Design review of the part built by this model. Coordinates are the model's own, in mm. A direction names the side the tool comes from. Coordinates: 2 decimals unless noted, no trailing zeros. Order: outer loops, then holes, each group sorted by start corner. A loop starts at its lowest first (then second) coordinate and runs counter-clockwise, first axis right, second up. Notation, with made-up numbers: M -16,13.5 L -7,13.5 A29 ccw -7,34.5 Z; hole C 57,63.25 d4. An arc over 180 degrees is marked long. Answer as a JSON object with one key per item and string values.
from build123d import *

# Parameters (mm, degrees)
SKETCH_1_W          = 60
SKETCH_1_H          = 80
EXTRUDE_1_DEPTH     = 5
SKETCH_2_W          = 40.5
SKETCH_2_H          = 20.5
CUT_EXTRUDE_1_DEPTH = 6
SKETCH_3_W          = 7
SKETCH_3_H          = 20.5
EXTRUDE_2_DEPTH     = 23
SKETCH_4_R          = 1.5
CUT_EXTRUDE_2_DEPTH = 10
FILLET_1_R          = 5
SKETCH_6_W          = 7
SKETCH_6_H          = 6.5
CUT_EXTRUDE_9_DEPTH = 23
FILLET_4_R          = 1
FILLET_6_R          = 1


with BuildPart() as part:
    # 草图1 → 凸台-拉伸1 (new body)
    with BuildSketch(Plane(origin=(0, 0, 0), x_dir=(1, 0, 0), z_dir=(0, 1, 0))):
        Rectangle(SKETCH_1_W, SKETCH_1_H)
    extrude(amount=EXTRUDE_1_DEPTH)

    # 草图2 → 切除-拉伸1 (cut, through all)
    with BuildSketch(Plane(origin=(0, 5, 0), x_dir=(1, 0, 0), z_dir=(0, 1, 0))):
        with Locations((0, -15)):
            Rectangle(SKETCH_2_W, SKETCH_2_H)
        with Locations((0, 15)):
            Rectangle(SKETCH_2_W, SKETCH_2_H)
    extrude(amount=-CUT_EXTRUDE_1_DEPTH, mode=Mode.SUBTRACT)

    # 草图3 → 凸台-拉伸2 (add)
    with BuildSketch(Plane(origin=(0, 5, 0), x_dir=(1, 0, 0), z_dir=(0, 1, 0))):
        with Locations((-23.75, 15)):
            Rectangle(SKETCH_3_W, SKETCH_3_H)
        with Locations((23.75, 15)):
            Rectangle(SKETCH_3_W, SKETCH_3_H)
        with Locations((23.75, -15)):
            Rectangle(SKETCH_3_W, SKETCH_3_H)
        with Locations((-23.75, -15)):
            Rectangle(SKETCH_3_W, SKETCH_3_H)
    extrude(amount=EXTRUDE_2_DEPTH)

    # 草图4 → 切除-拉伸2 (cut)
    with BuildSketch(Plane(origin=(0, 28, 0), x_dir=(1, 0, 0), z_dir=(0, 1, 0))):
        with Locations((-24.55, 20)):
            Circle(SKETCH_4_R)
        with Locations((-24.55, 10)):
            Circle(SKETCH_4_R)
        with Locations((24.55, 10)):
            Circle(SKETCH_4_R)
        with Locations((24.55, 20)):
            Circle(SKETCH_4_R)
        with Locations((24.55, -10)):
            Circle(SKETCH_4_R)
        with Locations((24.55, -20)):
            Circle(SKETCH_4_R)
        with Locations((-24.55, -10)):
            Circle(SKETCH_4_R)
        with Locations((-24.55, -20)):
            Circle(SKETCH_4_R)
    extrude(amount=-CUT_EXTRUDE_2_DEPTH, mode=Mode.SUBTRACT)

    # 圆角1
    fillet_1_edges = [part.edges().sort_by_distance(p)[0] for p in [
        (-30, 2.5, -40),
        (30, 2.5, -40),
        (30, 2.5, 40),
        (-30, 2.5, 40),
    ]]
    fillet(fillet_1_edges, radius=FILLET_1_R)

    # 草图6 → 切除-拉伸9 (cut)
    with BuildSketch(Plane(origin=(0, 28, 0), x_dir=(1, 0, 0), z_dir=(0, 1, 0))):
        with Locations((-23.75, 15)):
            Rectangle(SKETCH_6_W, SKETCH_6_H)
        with Locations((23.75, 15)):
            Rectangle(SKETCH_6_W, SKETCH_6_H)
        with Locations((23.75, -15)):
            Rectangle(SKETCH_6_W, SKETCH_6_H)
        with Locations((-23.75, -15)):
            Rectangle(SKETCH_6_W, SKETCH_6_H)
    extrude(amount=-CUT_EXTRUDE_9_DEPTH, mode=Mode.SUBTRACT)

    # 圆角4
    fillet_4_edges = [part.edges().sort_by_distance(p)[0] for p in [
        (-27.25, 16.5, 18.25),
        (-27.25, 16.5, 11.75),
        (27.25, 16.5, 11.75),
        (27.25, 16.5, 18.25),
        (27.25, 16.5, -18.25),
        (27.25, 16.5, -11.75),
        (-27.25, 16.5, -11.75),
        (-27.25, 16.5, -18.25),
        (-27.25, 16.5, -25.25),
        (-27.25, 16.5, -4.75),
        (27.25, 16.5, -4.75),
        (27.25, 16.5, -25.25),
        (27.25, 16.5, 25.25),
        (27.25, 16.5, 4.75),
        (-27.25, 16.5, 4.75),
        (-27.25, 16.5, 25.25),
    ]]
    fillet(fillet_4_edges, radius=FILLET_4_R)

    # 圆角6
    fillet_6_edges = [part.edges().sort_by_distance(p)[0] for p in [
        (-23.25, 5, 11.75),
        (23.25, 5, 18.25),
        (23.25, 5, -11.75),
        (-23.25, 5, -18.25),
        (23.25, 5, -25.25),
        (27.25, 5, -21.75),
        (23.25, 5, -18.25),
        (27.25, 5, -8.25),
        (23.25, 5, 4.75),
        (27.25, 5, 8.25),
        (23.25, 5, 11.75),
        (27.25, 5, 21.75),
        (-23.25, 5, 18.25),
        (-27.25, 5, 21.75),
        (-23.25, 5, 25.25),
        (-27.25, 5, 8.25),
        (-27.25, 5, -21.75),
        (-23.25, 5, -11.75),
        (-27.25, 5, -8.25),
        (-23.25, 5, -4.75),
        (26.957106781, 5, -24.957106781),
        (26.957106781, 5, -18.542893219),
        (26.957106781, 5, -11.457106781),
        (26.957106781, 5, -5.042893219),
        (26.957106781, 5, 5.042893219),
        (26.957106781, 5, 11.457106781),
        (26.957106781, 5, 18.542893219),
        (26.957106781, 5, 24.957106781),
        (-26.957106781, 5, 18.542893219),
        (-26.957106781, 5, 24.957106781),
        (-26.957106781, 5, 5.042893219),
        (-26.957106781, 5, 11.457106781),
        (-26.957106781, 5, -24.957106781),
        (-26.957106781, 5, -11.457106781),
        (-26.957106781, 5, -5.042893219),
        (-26.957106781, 5, -18.542893219),
        (-23.25, 5, -25.25),
        (23.25, 5, -4.75),
        (23.25, 5, 25.25),
        (-23.25, 5, 4.75),
    ]]
    fillet(fillet_6_edges, radius=FILLET_6_R)


solid = part.part
1) Mouldability with a two-part tool opening along X and no side actions: class faces 6 (the flat face through (-27.25, 17, 22)), 7 (the flat face through (-24, 28, -22)), 8 (the flat face through (20.25, 14, -10)) as released by +X, released by -X, zero draft, split by the parting line, or undercut.
Taken from the geometry:
{"face 6": "released by -X", "face 7": "zero draft", "face 8": "undercut"}
2) To check wall thickness, follow L1, parallel to Z at x = -23.5, y = 11; L2, parallel to X at y = 24, z = -20; L3, parallel to X at y = 3.25, z = -15.5. State the ranges of each line that lie inside material, in increasing order.
Taken from the geometry:
{"L1": "z = -25.25 to -18.25, -11.75 to -4.75, 4.75 to 11.75, 18.25 to 25.25", "L2": "x = -27.25 to -26.05, -23.05 to -20.25, 20.25 to 23.05, 26.05 to 27.25", "L3": "x = -30 to -20.25, 20.25 to 30"}
3) Add section B-B (y = 2.75). State the section outline as (x, z) points.
Taken from the geometry:
{"outline": "M -30,-35 A5 ccw -25,-40 L 25,-40 A5 ccw 30,-35 L 30,35 A5 ccw 25,40 L -25,40 A5 ccw -30,35 Z; hole M -20.25,-25.25 L 20.25,-25.25 L 20.25,-4.75 L -20.25,-4.75 Z; hole M -20.25,4.75 L 20.25,4.75 L 20.25,25.25 L -20.25,25.25 Z"}
4) Add section C-C (y = 22.25). Count the separate pieces of the cut face and the enclosed holes in it, and give its area (3 significant figures).
Taken from the geometry:
{"separate pieces": "8", "enclosed holes": "8", "area": "332 mm2"}
5) Tool access review of faces 1 (the flat face through (-25, 18, -20)), 2 (the flat face through (0, 3, -4.75)), 3 (the flat face through (-27.25, 17, 8)), 4 (the flat face through (-23, 17, -11.75)), 5 (the flat face through (23, 17, 25.25)): name each direction out of +Z, -Z, +X, -X, +Y, -Y from which nothing blocks a thin tool from reaching the whole face with its end or side.
Taken from the geometry:
{"face 1": "+Y", "face 2": "+Y, -Y", "face 3": "+Z, -Z, -X, +Y", "face 4": "+X, -X, +Y", "face 5": "+Z, +X, -X, +Y"}
6) Add section A-A (x = 13.5). State the section outline as (y, z) points, and give its area (3 significant figures).
Taken from the geometry:
{"outline": "M 0,-40 L 5,-40 L 5,-25.25 L 0,-25.25 Z; M 0,-4.75 L 5,-4.75 L 5,4.75 L 0,4.75 Z; M 0,25.25 L 5,25.25 L 5,40 L 0,40 Z", "area": "195 mm2"}
7) Insertion check: pin 1 Ø10 at (y, z) = (14, 25.5) entering from +X; pin 2 Ø4 at (y, z) = (22, 21.5) entering from -X; pin 3 Ø8 at (x, z) = (-13.5, 30) entering from -Y; pin 4 Ø5 at (x, y) = (-24.5, 16.5) entering from +Z. Each pin has a flat end and moves straight along its axis. Give the tip position at first contact, or say it passes through.
Taken from the geometry:
{"pin 1": "stops at x = 27.25", "pin 2": "stops at x = -27.25", "pin 3": "stops at y = 0", "pin 4": "stops at z = 25.25"}
